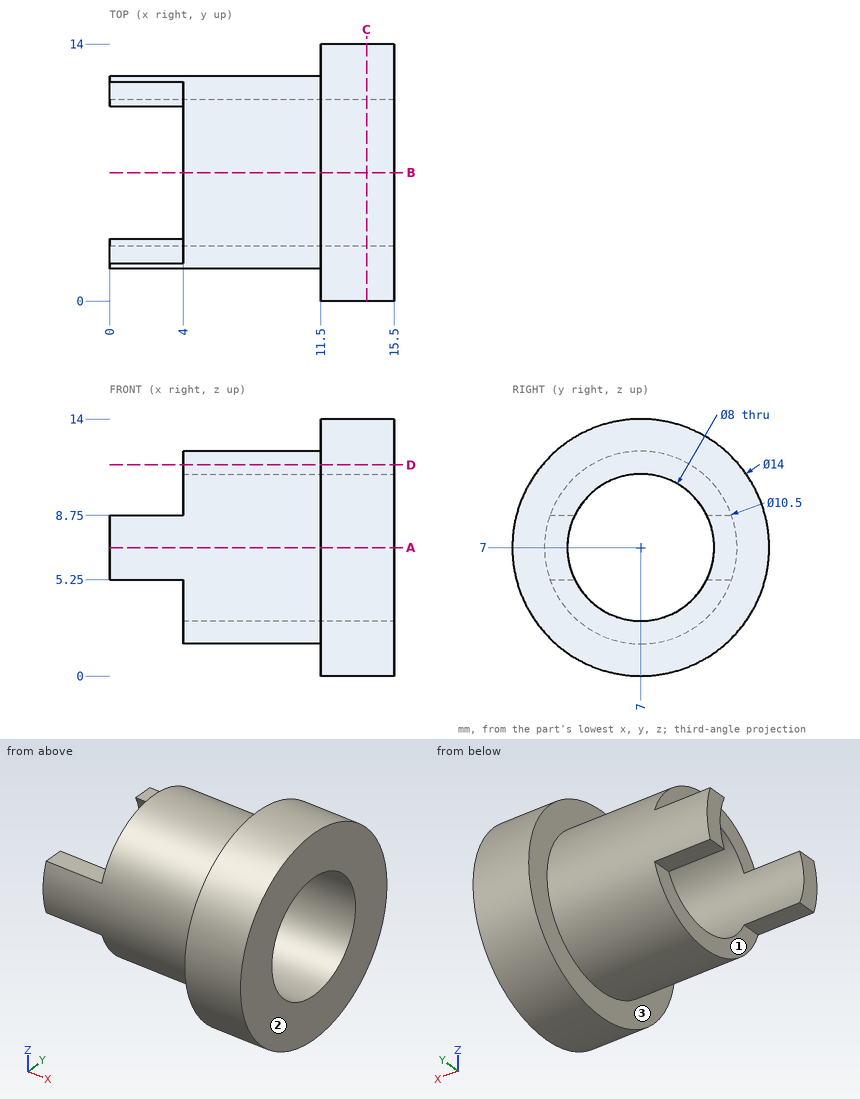
Geometry: see drawing. Coordinates: mm, zero at the bounding-box minimum. A direction names the side the tool comes from. Coordinates: 2 decimals unless noted, no trailing zeros. Loops run counter-clockwise (first coordinate to the right, second up) from the corner with the lowest first, then second, coordinate; pieces in that order, holes last. Notation, with made-up numbers: (29, 39) -> (61, 39) arc R18 cw to (61, 69) -> close; hole circle Ø7 at (2.5, 0). An arc over 180 degrees is marked (long way). Use a Markdown table: item, result.
1) Cut plane D-D (z = 11.5). Return the cut outline in (x, y), then the cut area to 3 significant figures.
Results found:
| item | result |
|---|---|
| outline | (4, 4.3) -> (11.5, 4.3) -> (11.5, 1.64) -> (15.5, 1.64) -> (15.5, 12.36) -> (11.5, 12.36) -> (11.5, 9.7) -> (4, 9.7) -> close |
| area | 83.5 mm2 |
2) Cut plane A-A (z = 7). Return the cut outline in (x, y).
Results found:
| item | result |
|---|---|
| outline | (0, 1.75) -> (11.5, 1.75) -> (11.5, 0) -> (15.5, 0) -> (15.5, 3) -> (0, 3) -> close; (0, 11) -> (15.5, 11) -> (15.5, 14) -> (11.5, 14) -> (11.5, 12.25) -> (0, 12.25) -> close |
3) Cut plane C-C (x = 14). Return the cut outline in (y, z).
Results found:
| item | result |
|---|---|
| outline | circle Ø14 at (7, 7); hole circle Ø8 at (7, 7) |
4) Contact query for flat-ended pins moving along their axis: pin 1 (1.1 mm diameter, centred on x = 2, y = 11.5, fed in from -Z); pin 2 (1.5 mm diameter, centred on y = 8.5, z = 8.5, fed in from -X); pin 3 (1.5 mm diameter, centred on x = 6, z = 6.5, fed in from -Y); pin 4 (6 mm diameter, centred on x = 2, z = 4.5, fed in from +Y). Output: stop coordinate, or through.
Results found:
| item | result |
|---|---|
| pin 1 | stops at z = 5.25 |
| pin 2 | passes through |
| pin 3 | stops at y = 1.75 |
| pin 4 | stops at y = 12.25 |
5) Material intervals for line 1 along Y through (x, z) = (4.75, 7); line 2 along X through (y, z) = (3, 4), sorted ascending. Write a range as from..to.
Results found:
| item | result |
|---|---|
| line 1 | y = 1.75..3, 11..12.25 |
| line 2 | x = 4..15.5 |
6) Access query for the marked faces 1, 2 and 3. Directions: +Z, -Z, +X, -X, +Y, -Y. A direction counts if a zero-diameter tool reaches every point of the face in a straight line with its end or side. Return the directions, or none.
Results found:
| item | result |
|---|---|
| face 1 | -Z, -X, +Y, -Y |
| face 2 | +Z, -Z, +X, +Y, -Y |
| face 3 | -X |
7) Cut plane B-B (y = 7). Return the cut outline in (x, z).
Results found:
| item | result |
|---|---|
| outline | (4, 1.75) -> (11.5, 1.75) -> (11.5, 0) -> (15.5, 0) -> (15.5, 3) -> (4, 3) -> close; (4, 11) -> (15.5, 11) -> (15.5, 14) -> (11.5, 14) -> (11.5, 12.25) -> (4, 12.25) -> close |
